```python
from build123d import *

# Parameters (mm, degrees)
CYLINDER012029001057_R       = 10
CYLINDER012029001057_DEPTH   = 3
BOX015001045_W               = 3
BOX015001045_H               = 12
BOX015001045_DEPTH           = 27
BOX015001045_PLACEMENT_ANGLE = 45
BOX015001046_W               = 3
BOX015001046_H               = 26
BOX015001046_DEPTH           = 76
BOX015001046_PLACEMENT_ANGLE = 45
BOX015001044_W               = 3
BOX015001044_H               = 39
BOX015001044_DEPTH           = 106
BOX015001042_W               = 3
BOX015001042_H               = 58
BOX015001042_DEPTH           = 100
FILLET004002003_R            = 2


with BuildPart() as cylinder012029001047:
    # Cylinder012029001057 → Cylinder012029001057 (new body)
    with BuildSketch(Plane(origin=(-279, 49.5, 32), x_dir=(0, 0, -1), z_dir=(1, 0, 0))):
        Circle(CYLINDER012029001057_R)
    extrude(amount=CYLINDER012029001057_DEPTH)


with BuildPart() as cube041:
    # Box015001045 → Box015001045 (new body)
    with BuildSketch(Plane.XY):
        with Locations((1.5, 6)):
            Rectangle(BOX015001045_W, BOX015001045_H)
    extrude(amount=BOX015001045_DEPTH)


with BuildPart() as cube041_1:
    # Box015001045 placement: moved
    add(cube041.part.moved(Location((-279, 84, 71))).rotate(Axis((-279, 84, 71), (1, 0, 0)), BOX015001045_PLACEMENT_ANGLE))


with BuildPart() as cube042:
    # Box015001046 → Box015001046 (new body)
    with BuildSketch(Plane.XY):
        with Locations((1.5, 13)):
            Rectangle(BOX015001046_W, BOX015001046_H)
    extrude(amount=BOX015001046_DEPTH)


with BuildPart() as cube042_1:
    # Box015001046 placement: moved
    add(cube042.part.moved(Location((-279, 33, -35))).rotate(Axis((-279, 33, -35), (1, 0, 0)), BOX015001046_PLACEMENT_ANGLE))


with BuildPart() as cube040:
    # Box015001044 → Box015001044 (new body)
    with BuildSketch(Plane(origin=(-279, 34, -16), x_dir=(1, 0, 0), z_dir=(0, 0, 1))):
        with Locations((1.5, 19.5)):
            Rectangle(BOX015001044_W, BOX015001044_H)
    extrude(amount=BOX015001044_DEPTH)


with BuildPart() as fillet004002003:
    # Box015001042 → Box015001042 (new body)
    with BuildSketch(Plane(origin=(-279, 0, 0), x_dir=(1, 0, 0), z_dir=(0, 0, 1))):
        with Locations((1.5, 29)):
            Rectangle(BOX015001042_W, BOX015001042_H)
    extrude(amount=BOX015001042_DEPTH)

    # Fusion001019007002: union Cube040
    add(cube040.part)

    # Cut003049: cut Cube042
    add(cube042_1.part, mode=Mode.SUBTRACT)

    # Cut003050: cut Cube041
    add(cube041_1.part, mode=Mode.SUBTRACT)

    # Cut003051: cut Cylinder012029001047
    add(cylinder012029001047.part, mode=Mode.SUBTRACT)

    # Fillet004002003
    fillet004002003_edges = [fillet004002003.edges().sort_by_distance(p)[0] for p in [
        (-277.5, 58, 90),
        (-277.5, 0, 34.769553),
        (-277.5, 50.769553, -16),
        (-277.5, 65, 90),
        (-277.5, 73, -16),
        (-277.5, 73, 82),
    ]]
    fillet(fillet004002003_edges, radius=FILLET004002003_R)


solid = fillet004002003.part
```
The listing builds one solid part. Answer for the finished solid, in the listing's coordinates (mm). A direction names the side the tool comes from. Give positions to 0.01 mm unless a question says otherwise; leave off trailing zeros. Write each loop counter-clockwise with the first axis right and the second up, starting at its lowest first coordinate (ties: lowest second). Pieces come first, ordered by that corner, then holes. Notation, with made-up numbers: (15, 80) -> (59, 80) arc R19 ccw to (59, 111) -> close; hole circle Ø10 at (81.25, 69.5). An arc over 180 degrees is marked (long way). Use one line per item in the form item = value.
1) For a pull along Z with two mould halves and no side action, classify faces 3 (the cylindrical face through (-277.52, 39.74, 34.17)), 4 (the flat face through (-278, 69, 86)), 5 (the flat face through (-276, 36, 54)) as +Z half, -Z half, draft (parallel to the pull), parting line (faces both ways), or undercut.
Result:
face_3 = undercut
face_4 = +Z half
face_5 = draft
2) Each of these flat-tipped pins is pushed along its axis until it touches: P1, Ø1.5, axis at x = -277, y = 61.5, coming from the +Z side; P2, Ø0.9, axis at x = -277, z = 98, coming from the +Y side. Where does it stop, or does it pass through?
Result:
P1 = 90
P2 = 58
3) Section A-A on x = -277.85 is taken. Write down the section's boundary in (y, z).
Result:
outline = (0, 35.6) arc R2 ccw to (0.59, 34.18) -> (50.18, -15.41) arc R2 ccw to (51.6, -16) -> (71, -16) arc R2 ccw to (73, -14) -> (73, 81.17) arc R2 ccw to (72.41, 82.59) -> (65.59, 89.41) arc R2 ccw to (64.17, 90) -> (60, 90) arc R2 cw to (58, 92) -> (58, 100) -> (0, 100) -> close; hole circle Ø20 at (49.5, 32)
4) Section D-D on z = 2 is taken. Write down the section's boundary in (x, y).
Result:
outline = (-279, 32.77) -> (-276, 32.77) -> (-276, 73) -> (-279, 73) -> close
5) Section C-C on y = 14.5 is taken. Write down the section's boundary in (x, z).
Result:
outline = (-279, 20.27) -> (-276, 20.27) -> (-276, 100) -> (-279, 100) -> close
6) Straight lines are drawn through the part: probe 1 along Y at (x, z) = (-278.35, 32); probe 2 along Z at (x, y) = (-277.7, 12.5); probe 3 along Z at (x, y) = (-278.2, 38). For each, find the intervals that lie inside material, in ascending order.
Result:
probe_1 = 2.77 to 39.5, 59.5 to 73
probe_2 = 22.27 to 100
probe_3 = -3.23 to 100
7) A tool of negligible diameter and unlimited length cuts with its end or side. For faces 1 (the flat face through (-278, 73, 33)), 2 (the flat face through (-278, 58, 96)), from which of +Z, -Z, +X, -X, +Y, -Y can it reach the whole face along a straight path? Write none if from no direction.
Result:
face_1 = +Z, -Z, +X, -X, +Y
face_2 = +Z, +X, -X, +Y
8) Section B-B on z = 31.5 is taken. Write down the section's boundary in (x, y).
Result:
outline = (-279, 3.27) -> (-276, 3.27) -> (-276, 39.51) -> (-279, 39.51) -> close; (-279, 59.49) -> (-276, 59.49) -> (-276, 73) -> (-279, 73) -> close
